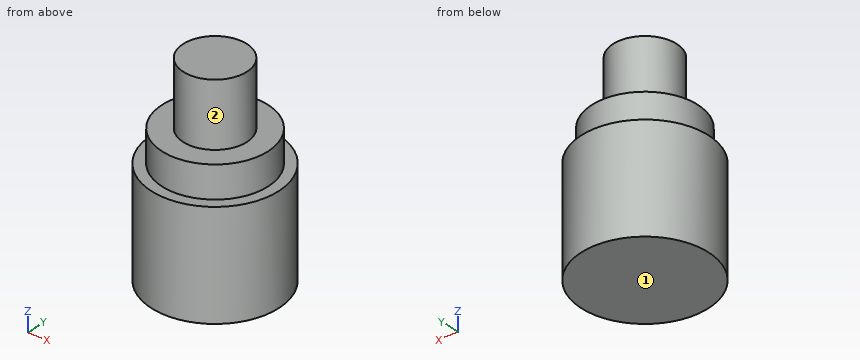
from build123d import *

# Parameters (mm, degrees)
SKETCH_1_R      = 30
EXTRUDE_1_DEPTH = 25
SKETCH_3_R      = 25
EXTRUDE_2_DEPTH = 15
SKETCH_4_R      = 15
EXTRUDE_3_DEPTH = 30


with BuildPart() as part:
    # 草图1 → 凸台-拉伸1 (new body, symmetric)
    with BuildSketch(Plane.XY):
        Circle(SKETCH_1_R)
    extrude(amount=EXTRUDE_1_DEPTH, both=True)

    # 草图3 → 凸台-拉伸2 (add)
    with BuildSketch(Plane.XY.offset(25)):
        Circle(SKETCH_3_R)
    extrude(amount=EXTRUDE_2_DEPTH)

    # 草图4 → 凸台-拉伸3 (add)
    with BuildSketch(Plane.XY.offset(40)):
        Circle(SKETCH_4_R)
    extrude(amount=EXTRUDE_3_DEPTH)


solid = part.part
CAD build for the part. Positions are in the model's coordinates, mm. Face numbers are marked on the shaded views. A direction names the side the tool comes from. Round coordinates to 2 decimals unless told otherwise and drop trailing zeros. Order: outer loops, then holes, each group sorted by start corner. A loop starts at its lowest first (then second) coordinate and runs counter-clockwise, first axis right, second up. Notation, with made-up numbers: (82.25, -17) -> (127.25, -17) arc R27 ccw to (127.25, 6) -> close; hole circle Ø3 at (42.5, -28). An arc over 180 degrees is marked (long way). Write each question's results on one line, items separated by ' | '.
1. Cut at C-C (z = 58.5). Give the cut face in (x, y).
Findings below:
outline: circle Ø30 at (0, 0)
2. 3-axis set-ups, long thin cutter, end or side, ignore diameter. For the marked faces 1 and 2: which of +Z, -Z, +X, -X, +Y, -Y reach the whole face in a straight line?
Findings below:
face 1: -Z, +X, -X, +Y, -Y | face 2: +Z
3. Wall check: line 1 along Z through (x, y) = (-14.5, -11.5); line 2 along X through (y, z) = (-24.5, -7); line 3 along Y through (x, z) = (2, 63). Give the ranges that are in metal, low to high. Write a range as [from, to].
Findings below:
line 1: z = [-25, 40] | line 2: x = [-17.31, 17.31] | line 3: y = [-14.87, 14.87]
4. Cut at A-A (x = 0). Give the cut face in (y, z), plus the area to 3 significant figures.
Findings below:
outline: (-30, -25) -> (30, -25) -> (30, 25) -> (25, 25) -> (25, 40) -> (15, 40) -> (15, 70) -> (-15, 70) -> (-15, 40) -> (-25, 40) -> (-25, 25) -> (-30, 25) -> close | area: 4,650 mm²
5. Flat gauge pins, fed straight in: P1, Ø8, axis at y = 13.5, z = -5, coming from the -X side; P2, Ø4, axis at y = -21, z = -8.5, coming from the +X side; P3, Ø2, axis at x = 17, y = 1, coming from the +Z side. Where does each tip first touch, or does it go through?
Findings below:
P1: stops at x = -28.46 | P2: stops at x = 23.22 | P3: stops at z = 40
6. Cut at D-D (y = 18.5). Give the cut face in (x, z).
Findings below:
outline: (-23.62, -25) -> (23.62, -25) -> (23.62, 25) -> (16.82, 25) -> (16.82, 40) -> (-16.82, 40) -> (-16.82, 25) -> (-23.62, 25) -> close
